```python
from build123d import *

# Parameters (mm, degrees)
BOSS_EXTRUDE1_DEPTH            = 15
CBORE_FOR_M3_SHCS1_D           = 3.4
CBORE_FOR_M3_SHCS1_CBORE_D     = 6.5
CBORE_FOR_M3_SHCS1_CBORE_DEPTH = 3
CUT_EXTRUDE1_REACH             = 92.43
BOSS_EXTRUDE2_DEPTH            = 1


with BuildPart() as part:
    # Sketch1 → Boss-Extrude1 (new body)
    with BuildSketch(Plane(origin=(0, 0, 0), x_dir=(1, 0, 0), z_dir=(0, 1, 0))):
        with BuildLine():
            Line((0, 0), (55.25, 0))
            Line((55.25, 0), (55.25, 55))
            ThreePointArc((55.25, 55), (50.856601718, 65.606601718), (40.25, 70))
            Line((40.25, 70), (15, 70))
            ThreePointArc((15, 70), (4.393398282, 65.606601718), (0, 55))
            Line((0, 55), (0, 0))
        make_face()
    extrude(amount=BOSS_EXTRUDE1_DEPTH)

    # CBORE for M3 SHCS1 (through all)
    with Locations(Plane(origin=(0, 15, 0), x_dir=(1, 0, 0), z_dir=(0, 1, 0))):
        with Locations((6, 34), (24, 34), (24, 6)):
            CounterBoreHole(CBORE_FOR_M3_SHCS1_D / 2, CBORE_FOR_M3_SHCS1_CBORE_D / 2, CBORE_FOR_M3_SHCS1_CBORE_DEPTH)

    # Sketch4 → Cut-Extrude1 (cut, up to next)
    with BuildSketch(Plane.ZY, mode=Mode.PRIVATE) as cut_extrude1_sk1:
        Polygon((-70, 0), (-45, 0), (-70, 7.5), align=None)
    cut_extrude1_tool1 = extrude(cut_extrude1_sk1.sketch, amount=-CUT_EXTRUDE1_REACH, mode=Mode.PRIVATE) & part.part
    add(cut_extrude1_tool1.solids().sort_by_distance((0, 2.5, -61.666667))[0], mode=Mode.SUBTRACT)

    # Sketch5 → Boss-Extrude2 (add)
    with BuildSketch(Plane(origin=(0, 15, 0), x_dir=(1, 0, 0), z_dir=(0, 1, 0))):
        with BuildLine():
            ThreePointArc((15, 70), (4.393398282, 65.606601718), (0, 55))
            Line((0, 55), (55.25, 55))
            ThreePointArc((55.25, 55), (50.856601718, 65.606601718), (40.25, 70))
            Line((40.25, 70), (15, 70))
        make_face()
    extrude(amount=BOSS_EXTRUDE2_DEPTH)


solid = part.part
```
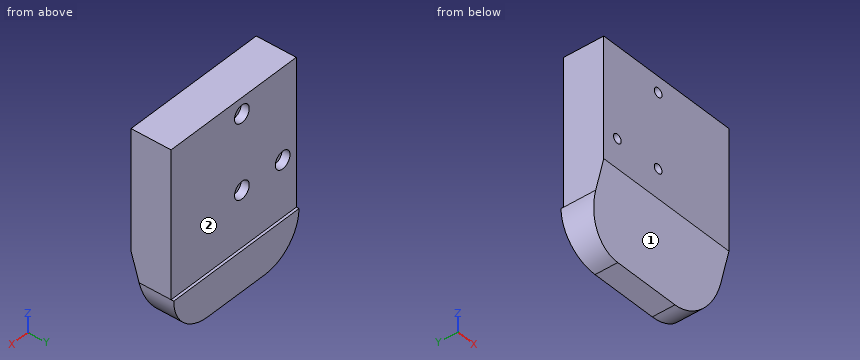
Model file for the job. Use its own axes, mm. Face numbers are marked on the shaded views. A direction names the side the tool comes from. Coordinates: 2 decimals unless noted, no trailing zeros. Order: outer loops, then holes, each group sorted by start corner. A loop starts at its lowest first (then second) coordinate and runs counter-clockwise, first axis right, second up. Notation, with made-up numbers: (-20, -21) - (15, -21) arc R30 cw to (15, 9) - close; hole circle Ø8 at (6, 70.25). An arc over 180 degrees is marked (long way). Return JSON: item names as keys, results as strings. Group by question number.
1) Saw through at D-D, the plane y = 8.5. Write the cut outline in (x, z), plus the area to 3 significant figures.
2) Tool access for the marked faces 1 and 2: list every direction of +Z, -Z, +X, -X, +Y, -Y with a clear straight run to the whole face (end or side of a thin tool).
3) Saw through at B-B, the plane z = -34. Write the cut outline in (x, y), plus the area to 3 significant figures.
4) Flat gauge pins, fed straight in: P1, Ø5, axis at x = 5.5, z = -34.5, coming from the +Y side; P2, Ø0.5, axis at x = 16, y = 15.5, coming from the +Z side; P3, Ø3, axis at x = 24, z = -6, coming from the +Y side; P4, Ø7, axis at x = 24, z = -34, coming from the +Y side. Where does each tip first touch, or does it go through?
5) Probe line 1 (X direction, y = 7.25, z = -34); line 2 (Z direction, x = 24, y = 14); line 3 (X direction, y = 14.2, z = -34). List the from-to ranges inside material, lowest first. Write a range as from..to.
6) Saw through at A-A, the plane x = 6. Write the cut outline in (y, z), plus the area to 3 significant figures.
7) Saw through at C-C, the plane z = -6. Write the cut outline in (x, y), plus the area to 3 significant figures.
Values found:
{
 "1": {"outline": "(0, -55) arc R15 ccw to (15, -70) - (40.25, -70) arc R15 ccw to (55.25, -55) - (55.25, 0) - (0, 0) - close; hole circle Ø3.4 at (6, -34); hole circle Ø3.4 at (24, -34); hole circle Ø3.4 at (24, -6)", "area": "3,740 mm²"},
 "2": {"face 1": "-Z, +X, -X, -Y", "face 2": "+Z, +X, -X, +Y"},
 "3": {"outline": "(0, 0) - (4.3, 0) - (4.3, 12) - (2.75, 12) - (2.75, 15) - (0, 15) - close; (7.7, 0) - (22.3, 0) - (22.3, 12) - (20.75, 12) - (20.75, 15) - (9.25, 15) - (9.25, 12) - (7.7, 12) - close; (25.7, 0) - (55.25, 0) - (55.25, 15) - (27.25, 15) - (27.25, 12) - (25.7, 12) - close", "area": "708 mm²"},
 "4": {"P1": "stops at y = 12", "P2": "stops at z = -55", "P3": "passes through", "P4": "stops at y = 15"},
 "5": {"line 1": "x = 0..4.3, 7.7..22.3, 25.7..55.25", "line 2": "z = -70..-37.25, -30.75..-9.25, -2.75..0", "line 3": "x = 0..2.75, 9.25..20.75, 27.25..55.25"},
 "6": {"outline": "(0, -45) - (6.6, -67) - (16, -67) - (16, -55) - (15, -55) - (15, -37.25) - (12, -37.25) - (12, -35.7) - (0, -35.7) - close; (0, -32.3) - (12, -32.3) - (12, -30.75) - (15, -30.75) - (15, 0) - (0, 0) - close", "area": "884 mm²"},
 "7": {"outline": "(0, 0) - (22.3, 0) - (22.3, 12) - (20.75, 12) - (20.75, 15) - (0, 15) - close; (25.7, 0) - (55.25, 0) - (55.25, 15) - (27.25, 15) - (27.25, 12) - (25.7, 12) - close", "area": "768 mm²"}
}
